The model under review builds one solid part; all positions refer to its coordinate system, in mm. A direction names the side the tool comes from. Coordinates: 2 decimals unless noted, no trailing zeros. Loops run counter-clockwise (first coordinate to the right, second up) from the corner with the lowest first, then second, coordinate; pieces in that order, holes last. Notation, with made-up numbers: M 8.5,49 L 51.5,49 A15 cw 51.5,57 Z; hole C 1,-27 d2. An arc over 180 degrees is marked long. Use one line per item in the form item = value.
```python
from build123d import *

# Parameters (mm, degrees)
SKETCH_1_W          = 75
SKETCH_1_H          = 45
EXTRUDE_1_DEPTH     = 18
SKETCH_2_W          = 71
SKETCH_2_H          = 41
CUT_EXTRUDE_1_DEPTH = 16
SKETCH_3_W          = 73
SKETCH_3_H          = 43
SKETCH_3_W_2        = 71
SKETCH_3_H_2        = 41
CUT_EXTRUDE_2_DEPTH = 3
FILLET_1_R          = 2
FILLET_2_R          = 1


with BuildPart() as part:
    # 草图1 → 凸台-拉伸1 (new body)
    with BuildSketch(Plane.XY):
        Rectangle(SKETCH_1_W, SKETCH_1_H)
    extrude(amount=EXTRUDE_1_DEPTH)

    # 草图2 → 切除-拉伸1 (cut)
    with BuildSketch(Plane.XY.offset(18)):
        Rectangle(SKETCH_2_W, SKETCH_2_H)
    extrude(amount=-CUT_EXTRUDE_1_DEPTH, mode=Mode.SUBTRACT)

    # 草图3 → 切除-拉伸2 (cut)
    with BuildSketch(Plane.XY.offset(18)):
        Rectangle(SKETCH_3_W, SKETCH_3_H)
        Rectangle(SKETCH_3_W_2, SKETCH_3_H_2, mode=Mode.SUBTRACT)
    extrude(amount=-CUT_EXTRUDE_2_DEPTH, mode=Mode.SUBTRACT)

    # 圆角1
    fillet_1_edges = [part.edges().sort_by_distance(p)[0] for p in [
        (-35.5, 20.5, 8.5),
        (35.5, 20.5, 8.5),
        (35.5, -20.5, 8.5),
        (-35.5, -20.5, 8.5),
        (-36.5, -21.5, 16.5),
        (-36.5, 21.5, 16.5),
        (36.5, 21.5, 16.5),
        (36.5, -21.5, 16.5),
        (-37.5, 22.5, 9),
        (37.5, 22.5, 9),
        (37.5, -22.5, 9),
        (-37.5, -22.5, 9),
    ]]
    fillet(fillet_1_edges, radius=FILLET_1_R)

    # 圆角2
    fillet_2_edges = [part.edges().sort_by_distance(p)[0] for p in [
        (0, -22.5, 0),
        (-37.5, 0, 0),
        (0, 22.5, 0),
        (37.5, 0, 0),
        (-36.914213562, 21.914213562, 0),
        (36.914213562, 21.914213562, 0),
        (36.914213562, -21.914213562, 0),
        (-36.914213562, -21.914213562, 0),
    ]]
    fillet(fillet_2_edges, radius=FILLET_2_R)


solid = part.part
```
1. Wall thickness on line 1 along X through (y, z) = (-11, 12); line 2 along Y through (x, z) = (-16, 15.5); line 3 along Y through (x, z) = (27, 12.5): over which ranges is each line inside the solid? List them lowest first. Write a range as from..to.
Response values:
line_1 = -37.5..-35.5, 35.5..37.5
line_2 = -22.5..-21.5, 21.5..22.5
line_3 = -22.5..-20.5, 20.5..22.5
2. Add section B-B (x = 28). State the section outline as (y, z) points.
Response values:
outline = M -22.5,1 A1 ccw -21.5,0 L 21.5,0 A1 ccw 22.5,1 L 22.5,18 L 21.5,18 L 21.5,15 L 20.5,15 L 20.5,2 L -20.5,2 L -20.5,15 L -21.5,15 L -21.5,18 L -22.5,18 Z
3. Add section A-A (z = 12.25). State the section outline as (x, y) points, then the cut area to 3 significant figures.
Response values:
outline = M -37.5,-20.5 A2 ccw -35.5,-22.5 L 35.5,-22.5 A2 ccw 37.5,-20.5 L 37.5,20.5 A2 ccw 35.5,22.5 L -35.5,22.5 A2 ccw -37.5,20.5 Z; hole M -35.5,-18.5 A2 ccw -33.5,-20.5 L 33.5,-20.5 A2 ccw 35.5,-18.5 L 35.5,18.5 A2 ccw 33.5,20.5 L -33.5,20.5 A2 ccw -35.5,18.5 Z
area = 464 mm^2
4. Machinability: for faces 1 (the face through (0, 21, 15)), 2 (the face through (0, -22.5, 9)), which of the approach directions +Z, -Z, +X, -X, +Y, -Y give a long, thin tool a straight path to every point of the face, cutting with its end or side? Answer none if there is none.
Response values:
face_1 = +Z
face_2 = +Z, -Z, +X, -X, -Y
5. Add section C-C (y = 6). State the section outline as (x, z) points.
Response values:
outline = M -37.5,1 A1 ccw -36.5,0 L 36.5,0 A1 ccw 37.5,1 L 37.5,18 L 36.5,18 L 36.5,15 L 35.5,15 L 35.5,2 L -35.5,2 L -35.5,15 L -36.5,15 L -36.5,18 L -37.5,18 Z
6. The part is to be moulded in two halves that separate along X. For faces 3 (the face through (36.9, -21.93, 9.62)), 4 (the face through (36.5, 0, 17)), 5 (the face through (0, 22.5, 9)), say which applies: pulls with the +X half, pulls with the -X half, needs draft (parallel to the pull), parting line crosses it, or undercut.
Response values:
face_3 = pulls with the +X half
face_4 = undercut
face_5 = needs draft
7. Insertion check: P1, Ø3, axis at x = 10.5, y = -12, coming from the +Z side. The pin has a flat end and moves straight along its axis. Give the tip position at first contact, or say it passes through.
Response values:
P1 = 2
